from build123d import *

# Parameters (mm, degrees)
BOSS_EXTRUDE1_START    = -34.925
SKETCH1_W              = 82.55
SKETCH1_H              = 81.407
BOSS_EXTRUDE1_DEPTH    = 3.175
SKETCH3_W              = 82.55
SKETCH3_H              = 3.175
BOSS_EXTRUDE2_DEPTH    = 50.8
F_10_CLEARANCE_HOLE2_D = 5.334
CHAMFER1_SIZE          = 3.175
FILLET2_R              = 3.937
SKETCH9_R              = 3.429
CUT_EXTRUDE2_DEPTH     = 54.975


with BuildPart() as part:
    # Sketch1 → Boss-Extrude1 (new body)
    with BuildSketch(Plane(origin=(0, 0, 0), x_dir=(1, 0, 0), z_dir=(0, 1, 0)).offset(BOSS_EXTRUDE1_START)):
        Rectangle(SKETCH1_W, SKETCH1_H)
    extrude(amount=BOSS_EXTRUDE1_DEPTH)

    # Sketch3 → Boss-Extrude2 (add)
    with BuildSketch(Plane(origin=(0, -31.75, 0), x_dir=(1, 0, 0), z_dir=(0, 1, 0))):
        with Locations((0, 39.116)):
            Rectangle(SKETCH3_W, SKETCH3_H)
    extrude(amount=BOSS_EXTRUDE2_DEPTH)

    # #10 Clearance Hole2 (through all)
    with Locations(Plane(origin=(0, 0, -40.7035), x_dir=(-1, 0, 0), z_dir=(0, 0, -1))):
        with Locations((22.225, 7.112), (9.525, 7.112), (-3.175, 7.112), (-15.875, 7.112), (-28.575, 7.112), (22.225, -18.288), (9.525, -18.288), (-3.175, -18.288), (-15.875, -18.288), (-28.575, -18.288), (34.925, 7.112), (34.925, -18.288), (-41.275, 7.112), (-41.275, -18.288)):
            Hole(F_10_CLEARANCE_HOLE2_D / 2)

    # Chamfer1
    chamfer1_edges = [part.edges().sort_by_distance(p)[0] for p in [
        (-41.275, 19.05, -39.116),
    ]]
    chamfer(chamfer1_edges, length=CHAMFER1_SIZE)

    # Fillet2
    fillet2_edges = [part.edges().sort_by_distance(p)[0] for p in [
        (0, -34.925, -40.7035),
    ]]
    fillet(fillet2_edges, radius=FILLET2_R)

    # Sketch9 → Cut-Extrude2 (cut, through all)
    with BuildSketch(Plane.XZ.offset(34.925)):
        with Locations((28.575, -24.8285)):
            Circle(SKETCH9_R)
        with Locations((28.575, 0.5715)):
            Circle(SKETCH9_R)
        with Locations((28.575, 25.9715)):
            Circle(SKETCH9_R)
        Polygon((-41.275, -37.5285), (-41.275, 40.7035), (15.875, 40.7035), align=None)
    extrude(amount=-CUT_EXTRUDE2_DEPTH, mode=Mode.SUBTRACT)


solid = part.part
Read the model definition and answer for the solid it produces. Units are mm, in the model's axes. A direction names the side the tool comes from. Give positions to 0.01 mm unless a question says otherwise; leave off trailing zeros. Write each loop counter-clockwise with the first axis right and the second up, starting at its lowest first coordinate (ties: lowest second). Pieces come first, ordered by that corner, then holes. Notation, with made-up numbers: M 89.5,43 L 125.5,43 A10 cw 125.5,54 Z; hole C 25.5,10.25 d3. An arc over 180 degrees is marked long. One line per item, written item: value. Start each with the question number.
(1) Determine the mould class of faces 1 (the flat face through (9, -34.925, -7)), 2 (the cylindrical face through (38.61, 7.17, -39.09)), 3 (the cylindrical face through (2.828, 9.756, -39.094)), 4 (the flat face through (-41.275, -10, -39)) for opening direction X: pulls with the +X half, pulls with the -X half, needs draft (parallel to the pull), parting line crosses it, or undercut.
(2) A tool of negligible diameter and unlimited length cuts with its end or side. For faces 5 (the flat face through (41.275, 14, -39)), 6 (the flat face through (-1, -7, -37.528)), from which of +Z, -Z, +X, -X, +Y, -Y can it reach the whole face along a straight path? Write none if from no direction.
(3) Find the intervals of material crossed by line 1 (Z direction, x = 26, y = -2.5); line 2 (Y direction, x = -10.5, z = -25) (3 decimals), in increasing order.
(4) Find section D-D (y = -3). Determine the outline of the cut face in (x, z) (1 decimal), plus the area to 3 significant figures.
(5) Find section A-A (x = -11). Give the number of separate pieces and of enclosed holes in the cut face, plus the area to 3 significant figures.
(6) Flat-ended cylindrical pins translate along their axes: pin 1 Ø4.5 at (x, y) = (-34.925, -18.288) entering from -Z; pin 2 Ø9 at (x, z) = (28.58, 25.97) entering from +Y; pin 3 Ø6 at (x, y) = (-34.925, 7.112) entering from +Z; pin 4 Ø11 at (x, z) = (28.58, 0.57) entering from -Y (3 decimals). Find the tip coordinate at first contact, or state that the pin passes through.
Results below:
1. face 1: needs draft
1. face 2: pulls with the +X half
1. face 3: undercut
1. face 4: pulls with the -X half
2. face 5: +Z, -Z, +X, +Y, -Y
2. face 6: +Z, +X, -X, +Y
3. line 1: z = -40.7 to -37.53
3. line 2: y = -34.925 to -31.75
4. outline: M -41.3,-40.7 L 41.3,-40.7 L 41.3,-37.5 L -41.3,-37.5 Z
4. area: 262 mm^2
5. separate pieces: 3
5. enclosed holes: 0
5. area: 271 mm^2
6. pin 1: passes through
6. pin 2: stops at y = -31.75
6. pin 3: stops at z = -37.53
6. pin 4: stops at y = -34.925
